from build123d import *

# Parameters (mm, degrees)
SKETCH_1_R      = 4
EXTRUDE_1_DEPTH = 16.7
FILLET_1_R      = 0.1
FILLET_2_R      = 0.1


with BuildPart() as part:
    # Эскиз1 → Бобышка-Вытянуть1 (new body)
    with BuildSketch(Plane(origin=(0, 0, 0), x_dir=(1, 0, 0), z_dir=(0, 1, 0))):
        Circle(SKETCH_1_R)
    extrude(amount=EXTRUDE_1_DEPTH)

    # Скругление1
    fillet_1_edges = [part.edges().sort_by_distance(p)[0] for p in [
        (-4, 16.7, 0),
    ]]
    fillet(fillet_1_edges, radius=FILLET_1_R)

    # Скругление2
    fillet_2_edges = [part.edges().sort_by_distance(p)[0] for p in [
        (-4, 0, 0),
    ]]
    fillet(fillet_2_edges, radius=FILLET_2_R)


solid = part.part
Geometry check sheet. Reference: the model listing, model coordinates, mm. Coordinates: 2 decimals unless noted, no trailing zeros. Order: outer loops, then holes, each group sorted by start corner. A loop starts at its lowest first (then second) coordinate and runs counter-clockwise, first axis right, second up. Notation, with made-up numbers: (-8, 14.5) - (15, 14.5) arc R20 ccw to (15, 30.5) - close; hole circle Ø1 at (-22.75, -22.5). An arc over 180 degrees is marked (long way). Answer in a Markdown table with one row per item. Add a question column.
1) Gauge pin test, flat end, axial feed: P1, Ø1, axis at x = -2.5, y = 12, coming from the -Z side. Record the tip position at first contact, or that the pin passes through.
2) Material ranges on line 1 along Z through (x, y) = (2.75, 10); line 2 along Z through (x, y) = (-3, 7.25); line 3 along X through (y, z) = (3.25, -1.25), recorded low to high. Write a range as [from, to].
3) Cross-section at A-A, the plane y = 9.75. Record the cut outline in (x, z), then the cut area to 3 significant figures.
Check result:
| question | item | result |
|---|---|---|
| 1 | P1 | stops at z = -3.46 |
| 2 | line 1 | z = [-2.9, 2.9] |
| 2 | line 2 | z = [-2.65, 2.65] |
| 2 | line 3 | x = [-3.8, 3.8] |
| 3 | outline | circle Ø8 at (0, 0) |
| 3 | area | 50.3 mm² |
